Read the model definition and answer for the solid it produces. Units are mm, in the model's axes. Coordinates: 2 decimals unless noted, no trailing zeros. Order: outer loops, then holes, each group sorted by start corner. A loop starts at its lowest first (then second) coordinate and runs counter-clockwise, first axis right, second up.
```python
from build123d import *

# Parameters (mm, degrees)
BOSS_EXTRUDE1_DEPTH              = 3.175
SKETCH2_R                        = 3.3655
CUT_EXTRUDE1_DEPTH               = 4.175
SKETCH8_W                        = 50.8
SKETCH8_H                        = 50.8
CUT_EXTRUDE9_DEPTH               = 4.175
FILLET2_R                        = 6.35
SKETCH9_W                        = 101.6
SKETCH9_H                        = 15.875
SKETCH9_W_2                      = 12.7
SKETCH9_H_2                      = 101.6
BOSS_EXTRUDE2_DEPTH              = 3.175
FILLET3_R                        = 3.175
SKETCH10_W                       = 31.75
SKETCH10_H                       = 15.875
CUT_EXTRUDE12_DEPTH              = 4.175
FILLET4_R                        = 6.35
F_17_64_0_26563_DIAMETER_HOLE1_D = 6.747002


with BuildPart() as part:
    # Sketch1 → Boss-Extrude1 (new body)
    with BuildSketch(Plane(origin=(0, 0, 0), x_dir=(0, 0, -1), z_dir=(1, 0, 0))):
        Polygon((0, 0), (0, -574.675), (31.75, -574.675), (257.175, -374.65), (257.175, 0), align=None)
    extrude(amount=BOSS_EXTRUDE1_DEPTH)

    # Sketch2 → Cut-Extrude1 (cut, through all)
    with BuildSketch(Plane(origin=(3.175, 0, 0), x_dir=(0, 0, -1), z_dir=(1, 0, 0))):
        with Locations((25.4, -561.975)):
            Circle(SKETCH2_R)
    extrude(amount=-CUT_EXTRUDE1_DEPTH, mode=Mode.SUBTRACT)

    # Sketch8 → Cut-Extrude9 (cut, through all)
    with BuildSketch(Plane(origin=(3.175, 0, 0), x_dir=(0, 0, -1), z_dir=(1, 0, 0))):
        with Locations((25.4, -279.4)):
            Rectangle(SKETCH8_W, SKETCH8_H)
    extrude(amount=-CUT_EXTRUDE9_DEPTH, mode=Mode.SUBTRACT)

    # Fillet2
    fillet2_edges = [part.edges().sort_by_distance(p)[0] for p in [
        (1.5875, -304.8, 0),
        (1.5875, -254, 0),
        (1.5875, -254, -50.8),
        (1.5875, -304.8, -50.8),
    ]]
    fillet(fillet2_edges, radius=FILLET2_R)

    # Sketch9 → Boss-Extrude2 (add)
    with BuildSketch(Plane(origin=(3.175, 0, 0), x_dir=(0, 0, -1), z_dir=(1, 0, 0))):
        with Locations((139.7, 7.9375)):
            Rectangle(SKETCH9_W, SKETCH9_H)
        with Locations((263.525, -101.6)):
            Rectangle(SKETCH9_W_2, SKETCH9_H_2)
        with Locations((263.525, -304.8)):
            Rectangle(SKETCH9_W_2, SKETCH9_H_2)
    extrude(amount=-BOSS_EXTRUDE2_DEPTH)

    # Fillet3
    fillet3_edges = [part.edges().sort_by_distance(p)[0] for p in [
        (1.5875, 0, -88.9),
        (1.5875, 15.875, -88.9),
        (1.5875, 15.875, -190.5),
        (1.5875, 0, -190.5),
        (1.5875, -152.4, -257.175),
        (1.5875, -50.8, -257.175),
        (1.5875, -50.8, -269.875),
        (1.5875, -152.4, -269.875),
        (1.5875, -355.6, -257.175),
        (1.5875, -254, -257.175),
        (1.5875, -254, -269.875),
        (1.5875, -355.6, -269.875),
    ]]
    fillet(fillet3_edges, radius=FILLET3_R)

    # Sketch10 → Cut-Extrude12 (cut, through all)
    with BuildSketch(Plane(origin=(3.175, 0, 0), x_dir=(0, 0, -1), z_dir=(1, 0, 0))):
        with Locations((15.875, -7.9375)):
            Rectangle(SKETCH10_W, SKETCH10_H)
    extrude(amount=-CUT_EXTRUDE12_DEPTH, mode=Mode.SUBTRACT)

    # Fillet4
    fillet4_edges = [part.edges().sort_by_distance(p)[0] for p in [
        (1.5875, -15.875, 0),
        (1.5875, 0, -31.75),
        (1.5875, -15.875, -31.75),
        (1.5875, 0, -257.175),
        (1.5875, -374.65, -257.175),
        (1.5875, -574.675, -31.75),
        (1.5875, -574.675, 0),
    ]]
    fillet(fillet4_edges, radius=FILLET4_R)

    # 17/64 (0.26563) Diameter Hole1 (through all)
    with Locations(Plane(origin=(3.175, 0, 0), x_dir=(0, 0, -1), z_dir=(1, 0, 0))):
        with Locations((244.475, -200.025)):
            Hole(F_17_64_0_26563_DIAMETER_HOLE1_D / 2)


solid = part.part
```
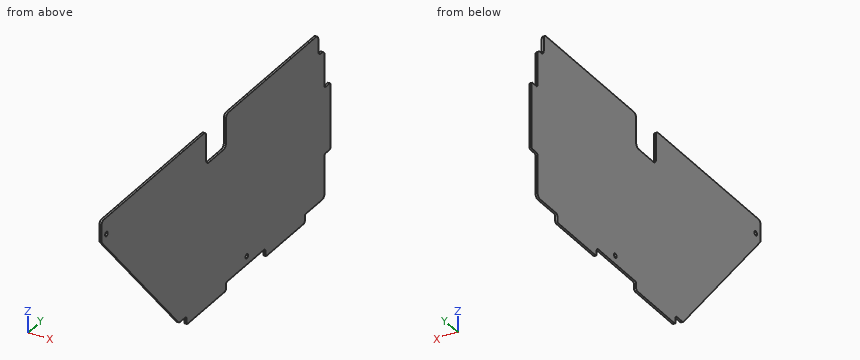
1) Straight lines are drawn through the part: line 1 (Y direction, x = 2.3, z = -25.4) (1 decimal); line 2 (Z direction, x = 1.9, y = -227) (3 decimals); line 3 (Z direction, x = 1.15, y = -293) (3 decimals). For each, find the intervals that lie inside material, in ascending order.
A:
line 1: y = -574.7 to -565.3, -558.6 to -304.8, -254 to -15.9
line 2: z = -257.175 to 0
line 3: z = -269.875 to -50.8
2) A cutting plane is placed at C-C, the plane z = -107. Determine the outline of the cut face in (x, y) (3 decimals), and give its area (3 significant figures).
A:
outline: (0, -507.904) - (3.175, -507.904) - (3.175, 15.875) - (0, 15.875) - close
area: 1,660 mm2
3) Flat-ended cylindrical pins translate along their axes: pin 1 Ø1.6 at (x, z) = (1, -264.5) entering from -Y; pin 2 Ø1 at (x, y) = (1.5, -30) entering from -Z (3 decimals); pin 3 Ø1 at (x, y) = (1.5, -284.5) entering from +Z. Find the tip coordinate at first contact, or state that the pin passes through.
A:
pin 1: stops at y = -355.6
pin 2: stops at z = -257.175
pin 3: stops at z = -50.8
4) A cutting plane is placed at A-A, the plane z = -59.5. Determine the outline of the cut face in (x, y) (3 decimals), and give its area (3 significant figures).
A:
outline: (0, -550.052) - (3.175, -550.052) - (3.175, 0) - (0, 0) - close
area: 1,750 mm2
5) A cutting plane is placed at B-B, the plane x = 1.5. State how many separate pieces and enclosed holes the cut face has, and give its area (3 significant figures).
A:
separate pieces: 1
enclosed holes: 2
area: 126,000 mm2
